Could you check a few things on this model? Use its own coordinates, in mm. Round coordinates to 2 decimals unless told otherwise and drop trailing zeros. Loops run counter-clockwise (first coordinate to the right, second up) from the corner with the lowest first, then second, coordinate; pieces in that order, holes last. Notation, with made-up numbers: (-12, 52.25) -> (44, 52.25) arc R13 ccw to (44, 69.25) -> close; hole circle Ø2 at (22, 25.25). An arc over 180 degrees is marked (long way). One line per item, written item: value.
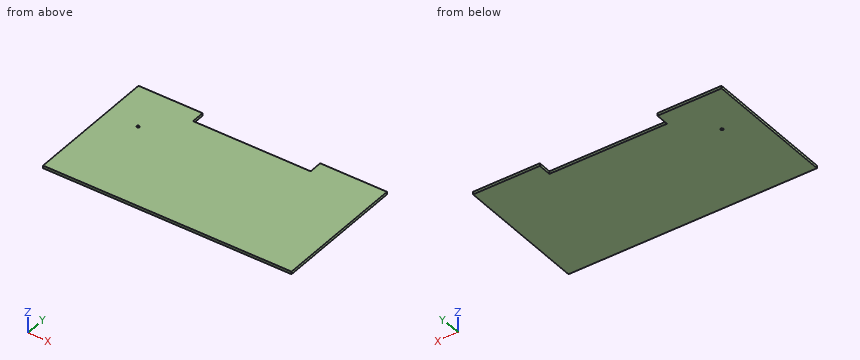
Autodesk Inventor part; units mm, degrees
ref_plane "YZ Plane" through (0, 0, 0) normal (1, 0, 0) x (0, 1, 0)
ref_plane "XZ Plane" through (0, 0, 0) normal (0, 1, 0) x (-1, 0, 0)
ref_plane "XY Plane" through (0, 0, 0) normal (0, 0, 1) x (1, 0, 0)
sketch "Sketch1" plane through (0, 0, 0) normal (0, 0, 1) x (1, 0, 0)
  line L0 (0, 0) -> (460, 0)
  line L1 (460, 0) -> (460, -250)
  line L2 (460, -250) -> (0, -250)
  line L3 (0, -250) -> (0, 0)
  line L4 (0, 0) -> (120, 0)
  line L5 (120, 0) -> (120, -25)
  line L6 (120, -25) -> (320, -25)
  line L7 (320, -25) -> (340, -25)
  line L8 (340, -25) -> (340, 0)
  line L9 (340, 0) -> (460, 0)
extrude "Extrusion1" add sketch "Sketch1" along normal blind 5 contours L0 L5 L6 L7 L8 L1 L2 L3
sketch "Sketch2" plane through (0, 0, 5) normal (0, 0, 1) x (1, 0, 0)
  circle A0 centre (60, -85) radius 2.5
  point P0 (0, 0)
extrude "Extrusion2" cut sketch "Sketch2" against normal through all
sketch "Sketch3" plane through (460, -250, 0) normal (1, 0, 0) x (0, 0, -1)
  line L0 (-5, 250) -> (-5, 0)
  line L1 (0, 0) -> (-5, 0)
  line L2 (-5, 250) -> (0, 250)
  line L3 (0, 250) -> (0, 0)
  line L4 (0, 0) -> (-5, 0)
  line L5 (-5, 0) -> (-5, 250)
extrude "Extrusion3" add sketch "Sketch3" along normal blind 5
sketch "Sketch4" plane through (0, 0, 5) normal (0, 0, 1) x (1, 0, 0)
  point P0 (0, 0)
sketch "Sketch5" plane through (465, -250, 0) normal (1, 0, 0) x (0, 0, -1)
  line L0 (0, 250) -> (-5, 250)
  line L1 (0, 250) -> (0, 0)
  line L2 (-5, 250) -> (0, 250)
  line L3 (0, 250) -> (0, 0)
  line L4 (0, 0) -> (-5, 0)
  line L5 (-5, 0) -> (-5, 250)
properties part number "new back support 2"
(1) If we section it at A-A, the plane z = 4.05: Please give me the cut outline in (x, y), then the cut area to 3 significant figures.
Recorded:
outline: (0, -250) -> (465, -250) -> (465, 0) -> (340, 0) -> (340, -25) -> (120, -25) -> (120, 0) -> (0, 0) -> close; hole circle Ø5 at (60, -85)
area: 111,000 mm²
(2) If I drill on L1, parallel to X at y = -21, z = 3.05; L2, parallel to Y at x = 229.5, z = 0.35; L3, parallel to Y at x = 60, z = 1.35, over which ranges is the centre line in solid material (lowest first)?
Recorded:
L1: 0 to 120, 340 to 465
L2: -250 to -25
L3: -250 to -87.5, -82.5 to 0
(3) If we section it at B-B, the plane x = 297.5: Please give me the cut outline in (y, z).
Recorded:
outline: (-250, 0) -> (-25, 0) -> (-25, 5) -> (-250, 5) -> close
(4) I'm going to push a flat-ended pin straight in: pin 1 Ø1 at (x, z) = (297, 4) entering from +Y. Where does the tip first touch, or does it pass through?
Recorded:
pin 1: y = -25
